from build123d import *

# Parameters (mm, degrees)
SKETCH1_W           = 35
SKETCH1_H           = 45
SKETCH1_R           = 1.1
BOSS_EXTRUDE1_DEPTH = 10
SKETCH5_W           = 35
SKETCH5_H           = 35
BOSS_EXTRUDE3_DEPTH = 10
CUT_EXTRUDE1_DEPTH  = 50
SKETCH7_W           = 23
SKETCH7_H           = 5
BOSS_EXTRUDE4_DEPTH = 10
SKETCH8_W           = 22.981157626
SKETCH8_H           = 5
BOSS_EXTRUDE5_DEPTH = 10
SKETCH9_W           = 12.018842374
SKETCH9_H           = 33
CUT_EXTRUDE2_DEPTH  = 40
SKETCH10_R          = 1
CUT_EXTRUDE3_DEPTH  = 10
SKETCH11_R          = 1
CUT_EXTRUDE4_DEPTH  = 10
SKETCH13_W          = 2.5
SKETCH13_H          = 10
CUT_EXTRUDE6_DEPTH  = 12.5
FILLET1_R           = 10
SKETCH14_R          = 2
CUT_EXTRUDE7_DEPTH  = 2.5


with BuildPart() as part:
    # Sketch1 → Boss-Extrude1 (new body)
    with BuildSketch(Plane(origin=(0, 0, 0), x_dir=(1, 0, 0), z_dir=(0, 1, 0))):
        with Locations((0, 17.5)):
            Rectangle(SKETCH1_W, SKETCH1_H)
        with Locations(Location((-10, -2.5, 0), (0, 0, 270))):
            Circle(SKETCH1_R, mode=Mode.SUBTRACT)
        with Locations(Location((10, -2.5, 0), (0, 0, 270))):
            Circle(SKETCH1_R, mode=Mode.SUBTRACT)
    extrude(amount=BOSS_EXTRUDE1_DEPTH)

    # Sketch5 → Boss-Extrude3 (add)
    with BuildSketch(Plane.XZ):
        with Locations((0, -22.5)):
            Rectangle(SKETCH5_W, SKETCH5_H)
    extrude(amount=BOSS_EXTRUDE3_DEPTH)

    # Sketch6 → Cut-Extrude1 (cut)
    with BuildSketch(Plane(origin=(17.5, 0, 0), x_dir=(0, 0, -1), z_dir=(1, 0, 0))):
        Polygon((5, -10), (40, 0), (40, -10), align=None)
    extrude(amount=-CUT_EXTRUDE1_DEPTH, mode=Mode.SUBTRACT)

    # Sketch7 → Boss-Extrude4 (add)
    with BuildSketch(Plane(origin=(0, 10, 0), x_dir=(1, 0, 0), z_dir=(0, 1, 0))):
        with Locations((-6, 37.5)):
            Rectangle(SKETCH7_W, SKETCH7_H)
    extrude(amount=BOSS_EXTRUDE4_DEPTH)

    # Sketch8 → Boss-Extrude5 (add)
    with BuildSketch(Plane(origin=(0, 10, 0), x_dir=(1, 0, 0), z_dir=(0, 1, 0))):
        with Locations((-6.009421187, 9.5)):
            Rectangle(SKETCH8_W, SKETCH8_H)
    extrude(amount=BOSS_EXTRUDE5_DEPTH)

    # Sketch9 → Cut-Extrude2 (cut)
    with BuildSketch(Plane(origin=(0, 10, 0), x_dir=(1, 0, 0), z_dir=(0, 1, 0))):
        with Locations((11.490578813, 23.5)):
            Rectangle(SKETCH9_W, SKETCH9_H)
    extrude(amount=-CUT_EXTRUDE2_DEPTH, mode=Mode.SUBTRACT)

    # Sketch10 → Cut-Extrude3 (cut)
    with BuildSketch(Plane(origin=(5.481157626, 0, 0), x_dir=(0, 0, -1), z_dir=(1, 0, 0))):
        with Locations((9.5, 16)):
            Circle(SKETCH10_R)
    extrude(amount=-CUT_EXTRUDE3_DEPTH, mode=Mode.SUBTRACT)

    # Sketch11 → Cut-Extrude4 (cut)
    with BuildSketch(Plane(origin=(5.5, 0, 0), x_dir=(0, 0, -1), z_dir=(1, 0, 0))):
        with Locations((37.5, 16)):
            Circle(SKETCH11_R)
    extrude(amount=-CUT_EXTRUDE4_DEPTH, mode=Mode.SUBTRACT)

    # Sketch13 → Cut-Extrude6 (cut)
    with BuildSketch(Plane.ZY.offset(17.5)):
        with Locations((-36.25, 15)):
            Rectangle(SKETCH13_W, SKETCH13_H)
    extrude(amount=-CUT_EXTRUDE6_DEPTH, mode=Mode.SUBTRACT)

    # Fillet1
    # the kernel refuses this fillet: 10 mm, written as the material it adds along each edge
    with BuildSketch(Plane(origin=(-5, -6.535945694, -37.5), x_dir=(-1, 0, 0), z_dir=(0, 1, 0))) as fillet1_piece_1_section:
        with BuildLine():
            CenterArc((6.614378278, 10), FILLET1_R, 228.590377891, 41.409622109)
            Line((0, 2.5), (0, 0))
            Line((0, 0), (6.614378278, 0))
        make_face()
    fillet1_piece_1 = extrude(amount=26.535945694, mode=Mode.PRIVATE)
    fillet1_piece_1 = split(fillet1_piece_1, bisect_by=Plane(origin=(-8.071773304, 0.306036312, -41.071127093), z_dir=(0, 0.9615239476408232, 0.27472112789737807)), keep=Keep.TOP, mode=Mode.PRIVATE)
    add(fillet1_piece_1)

    # Sketch14 → Cut-Extrude7 (cut)
    with BuildSketch(Plane(origin=(0, 10, 0), x_dir=(1, 0, 0), z_dir=(0, 1, 0))):
        with Locations(Location((10, -2.5, 0), (0, 0, 270))):
            Circle(SKETCH14_R)
        with Locations(Location((-10, -2.5, 0), (0, 0, 270))):
            Circle(SKETCH14_R)
    extrude(amount=-CUT_EXTRUDE7_DEPTH, mode=Mode.SUBTRACT)


solid = part.part
Could you check a few things on this model? Use its own coordinates, in mm. A direction names the side the tool comes from. Coordinates: 2 decimals unless noted, no trailing zeros. Loops run counter-clockwise (first coordinate to the right, second up) from the corner with the lowest first, then second, coordinate; pieces in that order, holes last.
1. Imagine slicing it at A-A (x = 10). Please give me the cut outline in (y, z).
2. We'd pull the mould along X, two halves only. Please class faces 1 (the face through (-4.5, 16, -37)), 2 (the face through (11.983, 8.768, 2.24)), 3 (the face through (-10.9, 7.5, 3.4)), 4 (the face through (0, -5, -5)): released by +X, released by -X, zero draft, split by the parting line, or undercut.
3. I need wall thicknesses on L1, parallel to X at y = 8.65, z = 2.5; L2, parallel to X at y = 3, z = 2.5; L3, parallel to Z at x = 10, y = 4.75. Which ranges of each line are inside material? Lowest first, please.
4. For P1, Ø4, axis at x = 9, z = -5, coming from the +Y side; P2, Ø8, axis at x = 8.5, z = 1, coming from the -Y side; P3, Ø10, axis at x = 3, z = -22.5, coming from the -Y side, each with a flat end and sliding along its axis, tell me the tip position at first contact or that it passes through.
5. Imagine slicing it at B-B (y = 16). Please give me the cut outline in (x, z).
6. For faces 5 (the face through (-6, 15, -12)), 6 (the face through (0, 0, 0)), 7 (the face through (-8.017, 8.768, 2.24)), 8 (the face through (-6, 15, -7)), 9 (the face through (0.57, 15.11, -37.96)), which set-ups out of +Z, -Z, +X, -X, +Y, -Y let a thin tool reach every point of the face, with its end or its side?
7. Imagine slicing it at C-C (z = 2.5). Please give me the cut outline in (x, y).
8. Imagine slicing it at D-D (x = 2). Please give me the cut outline in (y, z).
Computed values:
1. outline: (-10, -5) - (-9.43, -7) - (10, -7) - (10, 0.5) - (7.5, 0.5) - (7.5, 1.4) - (0, 1.4) - (0, -5) - close; (0, 3.6) - (7.5, 3.6) - (7.5, 4.5) - (10, 4.5) - (10, 5) - (0, 5) - close
2. face 1: released by +X
2. face 2: undercut
2. face 3: undercut
2. face 4: zero draft
3. L1: x = -17.5 to -12, -8 to 8, 12 to 17.5
3. L2: x = -17.5 to -11.1, -8.9 to 8.9, 11.1 to 17.5
3. L3: z = -7 to 1.4, 3.6 to 5
4. P1: stops at y = 10
4. P2: stops at y = 0
4. P3: stops at y = -6.43
5. outline: (-17.5, -40) - (5.5, -40) - (5.5, -38.5) - (-4.5, -38.5) - (-4.5, -36.5) - (5.5, -36.5) - (5.5, -35) - (-5, -35) arc R10 cw to (-11.61, -37.5) - (-17.5, -37.5) - close; (-17.5, -12) - (5.48, -12) - (5.48, -10.5) - (-4.52, -10.5) - (-4.52, -8.5) - (5.48, -8.5) - (5.48, -7) - (-17.5, -7) - close
6. face 5: +X, -X, +Y
6. face 6: +Z, +X, -X, -Y
6. face 7: +Y
6. face 8: +Z, +X, -X, +Y
6. face 9: +X
7. outline: (-17.5, 0) - (-11.1, 0) - (-11.1, 7.5) - (-12, 7.5) - (-12, 10) - (-17.5, 10) - close; (-8.9, 0) - (8.9, 0) - (8.9, 7.5) - (8, 7.5) - (8, 10) - (-8, 10) - (-8, 7.5) - (-8.9, 7.5) - close; (11.1, 0) - (17.5, 0) - (17.5, 10) - (12, 10) - (12, 7.5) - (11.1, 7.5) - close
8. outline: (-10, -5) - (0, -40) - (20, -40) - (20, -35) - (10, -35) - (10, -12) - (20, -12) - (20, -7) - (10, -7) - (10, 5) - (0, 5) - (0, -5) - close; hole circle Ø2 at (16, -37.5); hole circle Ø2 at (16, -9.5)
